Build history of the part. All positions in model axes, mm. A direction names the side the tool comes from. Coordinates: 2 decimals unless noted, no trailing zeros. Loops run counter-clockwise (first coordinate to the right, second up) from the corner with the lowest first, then second, coordinate; pieces in that order, holes last. Notation, with made-up numbers: (47.25, 15.5) - (85.25, 15.5) arc R21 ccw to (85.25, 28.5) - close; hole circle Ø9 at (-21, 27). An arc over 180 degrees is marked (long way). One line per item, written item: value.
```python
from build123d import *

# Parameters (mm, degrees)
F1_DEPTH = 14.2875


# Not quite as in the source:
# - a length typed as a fraction of an inch, garbled in the dataset ("3 / 203.2 mm" for 3/8 in), is restored


with BuildPart() as f1:
    # F0 (on Top) → F1 (new body)
    with BuildSketch(Plane.XY):
        with BuildLine():
            ThreePointArc((-0.0584694644, 41.0366132855), (-3.5379130554, 38.7889545067), (-6.4473585226, 35.840459168))
            ThreePointArc((-6.4473585226, 35.840459168), (-7.8691085687, 32.5448223466), (-7.4162920937, 28.9842672646))
            ThreePointArc((-7.4162920937, 28.9842672646), (-8.8119305122, 25.5953281623), (-8.2258973271, 21.977417171))
            ThreePointArc((-8.2258973271, 21.977417171), (-9.7181261566, 18.698842434), (-9.2097157612, 15.1327075437))
            ThreePointArc((-9.2097157612, 15.1327075437), (-10.6205392688, 11.8246856933), (-10.2093555033, 8.2519613206))
            Line((-10.2093555033, 8.2519613206), (-12.369341217, 7.1464567445))
            Line((-12.369341217, 7.1464567445), (-12.369341217, 4.6386048198))
            Line((-12.369341217, 4.6386048198), (-12.369341217, 4.5682978211))
            ThreePointArc((-12.369341217, 4.5682978211), (-15.5930977879, 3.1185654947), (-17.7027139134, 0.2823972963))
            ThreePointArc((-17.7027139134, 0.2823972963), (-21.0452825194, -1.0603738309), (-23.1384971151, -3.9919692741))
            ThreePointArc((-23.1384971151, -3.9919692741), (-26.5647165348, -5.2934051439), (-28.80180468, -8.19653302))
            ThreePointArc((-28.80180468, -8.19653302), (-32.1117440701, -9.5846599904), (-34.254974256, -12.4637500588))
            ThreePointArc((-34.254974256, -12.4637500588), (-35.4454588739, -16.4293701566), (-35.6585793197, -20.564340055))
            ThreePointArc((-35.6585793197, -20.564340055), (-31.9389059128, -22.4150036937), (-27.9142765499, -23.4461606411))
            ThreePointArc((-27.9142765499, -23.4461606411), (-24.3492963179, -23.0296138883), (-21.4921734029, -20.8571857766))
            ThreePointArc((-21.4921734029, -20.8571857766), (-17.8594468391, -20.3713745504), (-15.0192606046, -18.054899429))
            ThreePointArc((-15.0192606046, -18.054899429), (-11.4338171794, -17.7079201351), (-8.5996589687, -15.484556372))
            ThreePointArc((-8.5996589687, -15.484556372), (-5.0294162563, -15.0523544446), (-2.1409380715, -12.9098966718))
            Line((-2.1409380715, -12.9098966718), (0, -14.2561570176))
            Line((0, -14.2561570176), (1.9696742658, -12.9098966718))
            ThreePointArc((1.9696742658, -12.9098966718), (4.9392756736, -15.0084468105), (8.560301624, -15.3410370587))
            ThreePointArc((8.560301624, -15.3410370587), (11.3944598347, -17.5644008218), (14.9799032599, -17.9113801157))
            ThreePointArc((14.9799032599, -17.9113801157), (17.8200894944, -20.2278552371), (21.4528160582, -20.7136664634))
            ThreePointArc((21.4528160582, -20.7136664634), (24.3099389732, -22.886094575), (27.8749192052, -23.3026413279))
            ThreePointArc((27.8749192052, -23.3026413279), (31.8832272801, -22.3269581873), (35.5659238994, -20.4678624868))
            ThreePointArc((35.5659238994, -20.4678624868), (35.2059818343, -16.3418066269), (34.2156169113, -12.3202307456))
            ThreePointArc((34.2156169113, -12.3202307456), (32.0723867254, -9.4411406771), (28.7624473353, -8.0530137067))
            ThreePointArc((28.7624473353, -8.0530137067), (26.5253591901, -5.1498858306), (23.0991397704, -3.8484499608))
            ThreePointArc((23.0991397704, -3.8484499608), (21.0059251747, -0.9168545176), (17.6633565687, 0.4259166096))
            ThreePointArc((17.6633565687, 0.4259166096), (15.4847616458, 3.3168082822), (12.1560195839, 4.739132713))
            Line((12.1560195839, 4.739132713), (12.1560195839, 7.1464567445))
            Line((12.1560195839, 7.1464567445), (9.9960338703, 8.2519613206))
            ThreePointArc((9.9960338703, 8.2519613206), (10.4072176357, 11.8246856933), (8.9963941282, 15.1327075437))
            ThreePointArc((8.9963941282, 15.1327075437), (9.5048045235, 18.698842434), (8.012575694, 21.977417171))
            ThreePointArc((8.012575694, 21.977417171), (8.5986088792, 25.5953281623), (7.2029704606, 28.9842672646))
            ThreePointArc((7.2029704606, 28.9842672646), (7.6557869357, 32.5448223466), (6.2340368895, 35.840459168))
            ThreePointArc((6.2340368895, 35.840459168), (3.3823120514, 38.7952079886), (-0.0584694644, 41.0366132855))
        make_face()
    extrude(amount=F1_DEPTH)


solid = f1.part
```
Item 1: Drop flat-ended pins along their axis: P1, Ø3, axis at y = 3, z = 6.5, coming from the -X side; P2, Ø3, axis at x = -1.5, y = -10, coming from the -Z side; P3, Ø6, axis at y = -9, z = 11.5, coming from the +X side; P4, Ø3, axis at x = -18, z = 11, coming from the +Y side (3 decimals). Give the stop position or say it passes through.
Check result:
P1: stops at x = -17.06
P2: stops at z = 0
P3: stops at x = 34.08
P4: stops at y = 2.245
Item 2: Probe probe 1 along Y at (x, z) = (17, 13.75); probe 2 along Y at (x, z) = (1.5, 12); probe 3 along X at (y, z) = (36, 10). List the from-to ranges inside material, lowest first. Write a range as from..to.
Check result:
probe 1: y = -19.8..1.68
probe 2: y = -13.23..40.16
probe 3: x = -6.32..6.11
Item 3: Pull direction Y, two halves, no side cores. Call faces 1 (the face through (32.11, -9.47, 7.04)), 2 (the face through (17.772, -20.207, 7.044)), 3 (the face through (-7.86, 32.6, 7.04)), 4 (the face through (-8.806, 25.647, 7.044)): released by +Y, released by -Y, zero draft, split by the parting line, or undercut.
Check result:
face 1: released by +Y
face 2: released by -Y
face 3: undercut
face 4: undercut
Item 4: Cut at B-B, the plane y = 20.5. Write the cut outline in (x, z).
Check result:
outline: (-9.18, 0) - (8.97, 0) - (8.97, 14.29) - (-9.18, 14.29) - close
Item 5: Cut at A-A, the plane x = 30. Write the cut outline in (y, z).
Check result:
outline: (-22.91, 0) - (-8.33, 0) - (-8.33, 14.29) - (-22.91, 14.29) - close
Item 6: Tool access for faces 5 (the face through (0.971, -13.592, 7.044)), 6 (the face through (31.829, -22.347, 7.044)): list every direction of +Z, -Z, +X, -X, +Y, -Y with a clear straight run to the whole face (end or side of a thin tool).
Check result:
face 5: +Z, -Z, -Y
face 6: +Z, -Z, +X, -Y
